Geometry check sheet. Reference: the model listing, model coordinates, mm. A direction names the side the tool comes from. Coordinates: 2 decimals unless noted, no trailing zeros. Order: outer loops, then holes, each group sorted by start corner. A loop starts at its lowest first (then second) coordinate and runs counter-clockwise, first axis right, second up. Notation, with made-up numbers: M 8,-1 L 18,-1 A22 ccw 18,9 Z; hole C 0.5,73 d10. An arc over 180 degrees is marked long. Use CSV: the item, a comma, the result in double quotes. Start each with the question number.
```python
from build123d import *

# Parameters (mm, degrees)
SKETCH3_OUTSIDE_W                   = 54.458
SKETCH3_OUTSIDE_H                   = 54.458
SKETCH3_OUTSIDE_W_2                 = 20
SKETCH3_OUTSIDE_H_2                 = 34.409301068
CUT_EXTRUDE1_DEPTH                  = 10
CUT_EXTRUDE1_DEPTH_BACK             = 68
F_8_32_TAPPED_HOLE1_AT_2_COUNT      = 2
F_8_32_TAPPED_HOLE1_AT_2_PITCH      = 43.829214002
F_8_32_TAPPED_HOLE1_AT_3_COUNT      = 2
F_8_32_TAPPED_HOLE1_AT_3_PITCH      = 20
F_8_32_TAPPED_HOLE1_AT_4_COUNT      = 2
F_8_32_TAPPED_HOLE1_AT_4_PITCH      = 39
F_1_8_0_1250_DOWEL_HOLE1_AT_2_COUNT = 2
F_1_8_0_1250_DOWEL_HOLE1_AT_2_PITCH = 39
F_8_32_TAPPED_HOLE2_D               = 3.4544
F_8_32_TAPPED_HOLE2_DEPTH           = 10.71
F_8_32_TAPPED_HOLE2_TIP             = 1.037806461
CUT_EXTRUDE3_DEPTH                  = 1
CUT_EXTRUDE3_DEPTH_BACK             = 21


with BuildPart() as part:
    # Sketch2 → Revolve1 (revolve)
    with BuildSketch(Plane.XY):
        Polygon((-34, 0), (42, 0), (42, 4), (26, 4), (26, 6.7), (25, 6.7), (25, 17.204650534), (-25, 17.204650534), (-25, 6.7), (-27.5, 6.7), (-27.5, 4), (-34, 4), align=None)
    revolve(axis=Axis((-34, 0, 0), (1, 0, 0)))

    # Sketch3 outside → Cut-Extrude1 (cut, two sides)
    with BuildSketch(Plane.ZY.offset(25)) as cut_extrude1_sk:
        Rectangle(SKETCH3_OUTSIDE_W, SKETCH3_OUTSIDE_H)
        Rectangle(SKETCH3_OUTSIDE_W_2, SKETCH3_OUTSIDE_H_2, mode=Mode.SUBTRACT)
    extrude(amount=CUT_EXTRUDE1_DEPTH, mode=Mode.SUBTRACT)
    extrude(cut_extrude1_sk.sketch, amount=-CUT_EXTRUDE1_DEPTH_BACK, mode=Mode.SUBTRACT)

    # Sketch5 → #8-32 Tapped Hole1 (revolve, cut)
    with BuildSketch(Plane(origin=(19.5, 10, -10), x_dir=(0, 1, 0), z_dir=(1, 0, 0))):
        Polygon((0, 0), (0, 11.747806461), (1.7272, 10.71), (1.7272, 0), align=None)
    f_8_32_tapped_hole1 = revolve(axis=Axis((19.5, 10, -16.35), (0, 0, 1)), mode=Mode.SUBTRACT)

    # #8-32 Tapped Hole1 at 2: #8-32 Tapped Hole1 ×2
    with Locations(*[Vector(-0.889817463, -0.456316648, 0) * (i * F_8_32_TAPPED_HOLE1_AT_2_PITCH) for i in range(1, F_8_32_TAPPED_HOLE1_AT_2_COUNT)]):
        add(f_8_32_tapped_hole1, mode=Mode.SUBTRACT)

    # #8-32 Tapped Hole1 at 3: #8-32 Tapped Hole1 ×2
    with Locations(*[(0, -i * F_8_32_TAPPED_HOLE1_AT_3_PITCH, 0) for i in range(1, F_8_32_TAPPED_HOLE1_AT_3_COUNT)]):
        add(f_8_32_tapped_hole1, mode=Mode.SUBTRACT)

    # #8-32 Tapped Hole1 at 4: #8-32 Tapped Hole1 ×2
    with Locations(*[(-i * F_8_32_TAPPED_HOLE1_AT_4_PITCH, 0, 0) for i in range(1, F_8_32_TAPPED_HOLE1_AT_4_COUNT)]):
        add(f_8_32_tapped_hole1, mode=Mode.SUBTRACT)

    # Sketch7 → 1/8 (0.1250) Dowel Hole1 (revolve, cut)
    with BuildSketch(Plane(origin=(19.5, 0, -10), x_dir=(0, 1, 0), z_dir=(1, 0, 0))):
        Polygon((0, 0), (0, 6.953866233), (1.5875, 6), (1.5875, 0), align=None)
    f_1_8_0_1250_dowel_hole1 = revolve(axis=Axis((19.5, 0, -16.35), (0, 0, 1)), mode=Mode.SUBTRACT)

    # 1/8 (0.1250) Dowel Hole1 at 2: 1/8 (0.1250) Dowel Hole1 ×2
    with Locations(*[(-i * F_1_8_0_1250_DOWEL_HOLE1_AT_2_PITCH, 0, 0) for i in range(1, F_1_8_0_1250_DOWEL_HOLE1_AT_2_COUNT)]):
        add(f_1_8_0_1250_dowel_hole1, mode=Mode.SUBTRACT)

    # Mirror1: 1/8 (0.1250) Dowel Hole1, #8-32 Tapped Hole1 across plane
    add(f_1_8_0_1250_dowel_hole1.mirror(Plane.XY), mode=Mode.SUBTRACT)
    add(f_8_32_tapped_hole1.mirror(Plane.XY), mode=Mode.SUBTRACT)

    # Mirror1 copy 1 sketch → Mirror1 copy 1 (revolve, cut)
    with BuildSketch(Plane(origin=(-19.5, 0, 10), x_dir=(0, 1, 0), z_dir=(1, 0, 0))):
        Polygon((0, 0), (0, -6.953866233), (1.5875, -6), (1.5875, 0), align=None)
    revolve(axis=Axis((-19.5, 0, 16.35), (0, 0, 1)), mode=Mode.SUBTRACT)

    # Mirror1 copy 2 sketch → Mirror1 copy 2 (revolve, cut)
    with BuildSketch(Plane(origin=(-19.5, -10, 10), x_dir=(0, 1, 0), z_dir=(1, 0, 0))):
        Polygon((0, 0), (0, -11.747806461), (1.7272, -10.71), (1.7272, 0), align=None)
    revolve(axis=Axis((-19.5, -10, 16.35), (0, 0, 1)), mode=Mode.SUBTRACT)

    # Mirror1 copy 3 sketch → Mirror1 copy 3 (revolve, cut)
    with BuildSketch(Plane(origin=(19.5, -10, 10), x_dir=(0, 1, 0), z_dir=(1, 0, 0))):
        Polygon((0, 0), (0, -11.747806461), (1.7272, -10.71), (1.7272, 0), align=None)
    revolve(axis=Axis((19.5, -10, 16.35), (0, 0, 1)), mode=Mode.SUBTRACT)

    # Mirror1 copy 4 sketch → Mirror1 copy 4 (revolve, cut)
    with BuildSketch(Plane(origin=(-19.5, 10, 10), x_dir=(0, 1, 0), z_dir=(1, 0, 0))):
        Polygon((0, 0), (0, -11.747806461), (1.7272, -10.71), (1.7272, 0), align=None)
    revolve(axis=Axis((-19.5, 10, 16.35), (0, 0, 1)), mode=Mode.SUBTRACT)

    # #8-32 Tapped Hole2
    with Locations(Plane.ZY.offset(34)):
        with Locations((0, 0)):
            Hole(F_8_32_TAPPED_HOLE2_D / 2, depth=F_8_32_TAPPED_HOLE2_DEPTH)
            with Locations((0, 0, -(F_8_32_TAPPED_HOLE2_DEPTH + F_8_32_TAPPED_HOLE2_TIP / 2))):  # 118° drill point
                Cone(0, F_8_32_TAPPED_HOLE2_D / 2, F_8_32_TAPPED_HOLE2_TIP, mode=Mode.SUBTRACT)

    # Sketch12 → Cut-Extrude3 (cut, two sides)
    with BuildSketch(Plane.XY.offset(10)) as cut_extrude3_sk:
        with BuildLine():
            Line((-12.9125, -4.204650534), (12.9125, -4.204650534))
            ThreePointArc((12.9125, -4.204650534), (15.740927125, -3.033077659), (16.9125, -0.204650534))
            Line((16.9125, -0.204650534), (16.9125, 5))
            ThreePointArc((16.9125, 5), (15.740927125, 7.828427125), (12.9125, 9))
            Line((12.9125, 9), (-12.9125, 9))
            ThreePointArc((-12.9125, 9), (-15.740927125, 7.828427125), (-16.9125, 5))
            Line((-16.9125, 5), (-16.9125, -0.204650534))
            ThreePointArc((-16.9125, -0.204650534), (-15.740927125, -3.033077659), (-12.9125, -4.204650534))
        make_face()
        with BuildLine():
            Line((-12.9125, -9.204650534), (12.9125, -9.204650534))
            ThreePointArc((12.9125, -9.204650534), (15.740927125, -10.376223409), (16.9125, -13.204650534))
            Line((16.9125, -13.204650534), (16.9125, -17.204650534))
            Line((16.9125, -17.204650534), (-16.9125, -17.204650534))
            Line((-16.9125, -17.204650534), (-16.9125, -13.204650534))
            ThreePointArc((-16.9125, -13.204650534), (-15.740927125, -10.376223409), (-12.9125, -9.204650534))
        make_face()
    extrude(amount=CUT_EXTRUDE3_DEPTH, mode=Mode.SUBTRACT)
    extrude(cut_extrude3_sk.sketch, amount=-CUT_EXTRUDE3_DEPTH_BACK, mode=Mode.SUBTRACT)


solid = part.part
```
1) Draft check along Y on faces 1 (the face through (33.888, -0.867, -3.905)), 2 (the face through (15.71, -10.345, 0.14)), 3 (the face through (16.912, 2, 0)). Enter one of: +Y half, -Y half, draft (parallel to the pull), parting line (faces both ways), or undercut.
2) Section check B-B on x = -8. Record the boundary of the cut face in (y, z).
3) Section check D-D on x = 23.5. Record the boundary of the cut face in (y, z), then the cut area to 3 significant figures.
4) Material ranges on line 1 along X through (y, z) = (10, 2); line 2 along Y through (x, z) = (19.5, 0); line 3 along X through (y, z) = (0, -6.05), recorded low to high.
5) Section check C-C on y = -10. Record the boundary of the cut face in (x, z), then the cut area to 3 significant figures.
6) Set-up check for faces 4 (the face through (0, 9, 0)), 5 (the face through (-15.772, -10.407, 0.14)), 6 (the face through (26, -3, -3)): record each of +Z, -Z, +X, -X, +Y, -Y from which the full face is reachable in a straight line by a thin tool's end or side.
7) Gauge pin test, flat ends, axial feed: P1, Ø4, axis at y = 8, z = -5, coming from the +X side; P2, Ø2, axis at y = -10.5, z = 1, coming from the -X side; P3, Ø6, axis at y = -7.5, z = -3, coming from the -X side. Record the tip position at first contact, or that the pin passes through.
8) Section check A-A on y = 10. Record the boundary of the cut face in (x, z), then the cut area to 3 significant figures.
Results are:
1,face 1,"parting line"
1,face 2,"-Y half"
1,face 3,"undercut"
2,outline,"M -9.2,-10 L -4.2,-10 L -4.2,10 L -9.2,10 Z; M 9,-10 L 14,-10 A17.2 ccw 14,10 L 9,10 Z"
3,outline,"M -14,-10 L 14,-10 A17.2 ccw 14,10 L -14,10 A17.2 ccw Z"
3,area,"647 mm²"
4,line 1,"x = -25 to -21.23, -17.77 to 17.77, 21.23 to 25"
4,line 2,"y = -17.2 to -11.73, -8.27 to 8.27, 11.73 to 17.2"
4,line 3,"x = -27.5 to -21.09, -17.91 to -16.91, 16.91 to 17.91, 21.09 to 26"
5,outline,"M -25,-10 L -21.23,-10 L -21.23,10 L -25,10 Z; M -17.77,-10 L -15.31,-10 L -15.31,10 L -17.77,10 Z; M 15.31,-10 L 17.77,-10 L 17.77,10 L 15.31,10 Z; M 21.23,-10 L 25,-10 L 25,10 L 21.23,10 Z"
5,area,"250 mm²"
6,face 4,"+Z, -Z"
6,face 5,"+Z, -Z, -Y"
6,face 6,"+X"
7,P1,"stops at x = 25"
7,P2,"stops at x = -25"
7,P3,"stops at x = -27.5"
8,outline,"M -25,-10 L -21.23,-10 L -21.23,10 L -25,10 Z; M -17.77,-10 L 17.77,-10 L 17.77,10 L -17.77,10 Z; M 21.23,-10 L 25,-10 L 25,10 L 21.23,10 Z"
8,area,"862 mm²"
